Check sheet for the drawn part. Datum: minimum x, y, z corner. Units: mm. Coordinates: 2 decimals unless noted, no trailing zeros. Write each loop counter-clockwise with the first axis right and the second up, starting at its lowest first coordinate (ties: lowest second). Pieces come first, ordered by that corner, then holes. Notation, with made-up numbers: M -37,-9.75 L 10,-9.75 A20 ccw 10,-2.75 Z; hole C -36,10.25 d6. An arc over 180 degrees is marked long. Answer in a Markdown table with one row per item.
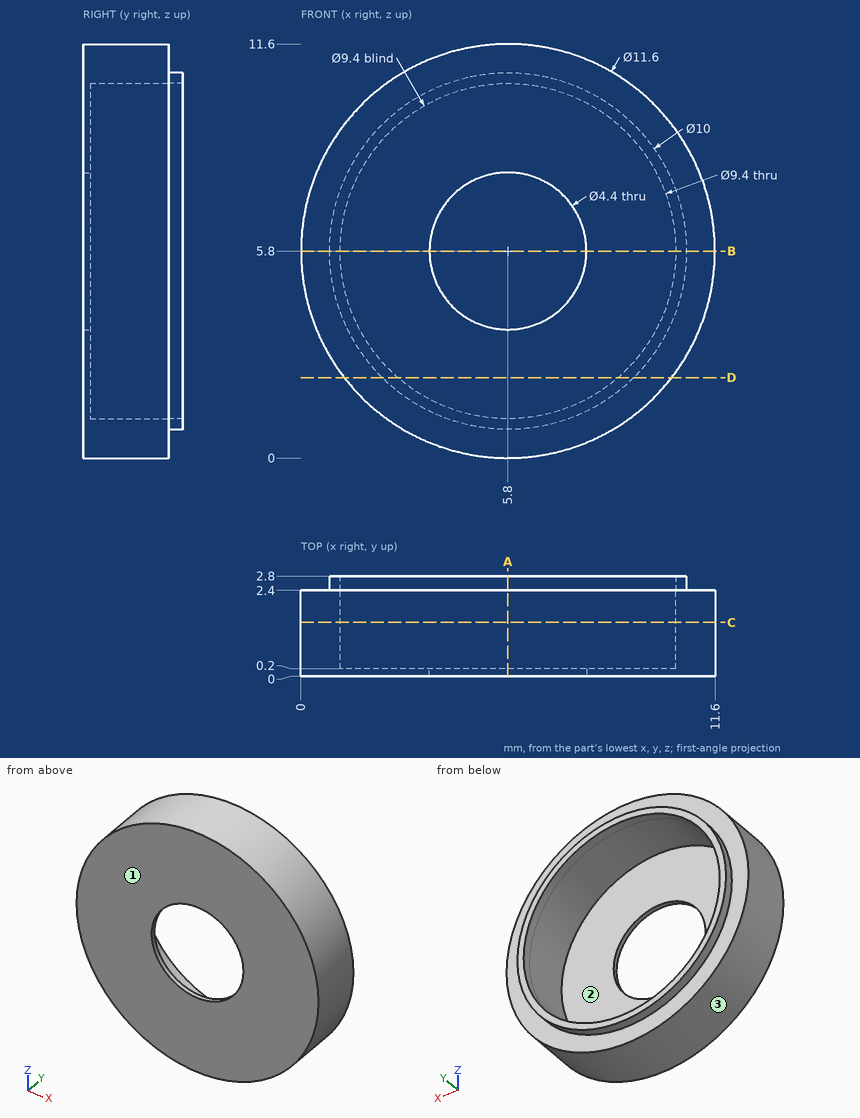
1) Sectioned sample at D-D (z = 2.25). Record the cut outline in (x, y).
Response values:
| item | result |
|---|---|
| outline | M 1.21,0 L 10.39,0 L 10.39,2.4 L 9.32,2.4 L 9.32,2.8 L 8.88,2.8 L 8.88,0.2 L 2.72,0.2 L 2.72,2.8 L 2.28,2.8 L 2.28,2.4 L 1.21,2.4 Z |
2) Sectioned sample at C-C (y = 1.5). Record the cut outline in (x, z).
Response values:
| item | result |
|---|---|
| outline | C 5.8,5.8 d11.6; hole C 5.8,5.8 d9.4 |
3) Depth check by flat-ended pin: pin 1 (2 mm diameter, centred on x = 5.5, z = 7.5, fed in from +Y); pin 2 (1 mm diameter, centred on y = 1, z = 6.5, fed in from -X); pin 3 (1.5 mm diameter, centred on y = 1, z = 2.5, fed in from -X). Enter the tip coordinate at first touch or a pass-through.
Response values:
| item | result |
|---|---|
| pin 1 | stops at y = 0.2 |
| pin 2 | stops at x = 0 |
| pin 3 | stops at x = 0.59 |
4) Sectioned sample at B-B (z = 5.8). Record the cut outline in (x, y).
Response values:
| item | result |
|---|---|
| outline | M 0,0 L 3.6,0 L 3.6,0.2 L 1.1,0.2 L 1.1,2.8 L 0.8,2.8 L 0.8,2.4 L 0,2.4 Z; M 8,0 L 11.6,0 L 11.6,2.4 L 10.8,2.4 L 10.8,2.8 L 10.5,2.8 L 10.5,0.2 L 8,0.2 Z |
5) Sectioned sample at A-A (x = 5.8). Record the cut outline in (y, z).
Response values:
| item | result |
|---|---|
| outline | M 0,0 L 2.4,0 L 2.4,0.8 L 2.8,0.8 L 2.8,1.1 L 0.2,1.1 L 0.2,3.6 L 0,3.6 Z; M 0,8 L 0.2,8 L 0.2,10.5 L 2.8,10.5 L 2.8,10.8 L 2.4,10.8 L 2.4,11.6 L 0,11.6 Z |
6) Release check for a two-part mould opening along Z. For the marked faces 1, 2 and 3 record: +Z half, -Z half, draft (parallel to the pull), parting line (faces both ways), or undercut.
Response values:
| item | result |
|---|---|
| face 1 | draft |
| face 2 | undercut |
| face 3 | parting line |
7) Thickness scan on L1, parallel to Z at x = 5.8, y = 1.4; L2, parallel to Z at x = 5.8, y = 0.1; L3, parallel to X at y = 1.05, z = 9.5. Record the ranges inside material, lowest first. Write a range as [from, to].
Response values:
| item | result |
|---|---|
| L1 | z = [0, 1.1], [10.5, 11.6] |
| L2 | z = [0, 3.6], [8, 11.6] |
| L3 | x = [1.33, 2.9], [8.7, 10.27] |
